Read the model definition and answer for the solid it produces. Units are mm, in the model's axes. A direction names the side the tool comes from. Coordinates: 2 decimals unless noted, no trailing zeros. Loops run counter-clockwise (first coordinate to the right, second up) from the corner with the lowest first, then second, coordinate; pieces in that order, holes last. Notation, with made-up numbers: (50.25, 9) -> (71.25, 9) arc R6 ccw to (71.25, 14) -> close; hole circle Ø8 at (82.25, 38.5). An arc over 180 degrees is marked (long way). Answer as a JSON object with one key per item and string values. Group by question number.
Q1. Straight lines are drawn through the part: line 1 along X through (y, z) = (-15, 187); line 2 along X through (y, z) = (-0.5, 65.5); line 3 along Y through (x, z) = (12, 143). For each, find the intervals that lie inside material, in ascending order. Write a range as [from, to].
Q2. The part is cut by section B-B on z = 196.5. State how many separate pieces and enclosed holes the cut face has, and give its area (3 significant figures).
Q3. Determine the mould class of faces 1 (the flat face through (45, -13, 125)), 2 (the cylindrical face through (41.5, -19.07, 125.22)) for opening direction Y: released by +Y, released by -Y, zero draft, split by the parting line, or undercut.
Q4. Each of these flat-tipped pins is pushed along its axis until it touches: P1, Ø1.5, axis at x = 21.5, y = -9, coming from the +Z side; P2, Ø2.5, axis at x = 24.5, z = 188.5, coming from the -Y side; P3, Ø4, axis at x = -34.5, y = -10.5, coming from the +Z side. Where does it stop, or does it pass through?
Q5. The part is cut by section A-A on x = 6. Write down the section's boundary in (y, z).
Q6. For faces 3 (the flat face through (-43, -4.1, 125)), 4 (the flat face through (43, -4.1, 125)), 5 (the flat face through (15.5, 0, 125)), determine the directions among +Z, -Z, +X, -X, +Y, -Y from which every point of the face is accessible in a straight line to the end or side of a thin tool.
from build123d import *

# Parameters (mm, degrees)
BOSS_EXTRUDE1_DEPTH = 254


with BuildPart() as part:
    # Sketch1 → Boss-Extrude1 (new body)
    with BuildSketch(Plane(origin=(0, 0, 0), x_dir=(-1, 0, 0), z_dir=(0, 0, -1))):
        Polygon((-26.6, 22.5), (-45, 22.5), (-45, 4.1), (-40.5, 4.1), (-40.5, 6.8), (-32, 6.8), (-29.7, 4.5), (-29.7, -4.5), (-32, -6.8), (-40.5, -6.8), (-40.5, -4.1), (-45, -4.1), (-45, -22.5), (-26.6, -22.5), (-26.6, -18), (-29.3, -18), (-29.3, -9.5), (-27, -7.2), (-18, -7.2), (-15.7, -9.5), (-15.7, -18), (-18.4, -18), (-18.4, -22.5), (18.4, -22.5), (18.4, -18), (15.7, -18), (15.7, -9.5), (18, -7.2), (27, -7.2), (29.3, -9.5), (29.3, -18), (26.6, -18), (26.6, -22.5), (45, -22.5), (45, -4.1), (40.5, -4.1), (40.5, -6.8), (32, -6.8), (29.7, -4.5), (29.7, 4.5), (32, 6.8), (40.5, 6.8), (40.5, 4.1), (45, 4.1), (45, 22.5), (26.6, 22.5), (26.6, 18), (29.3, 18), (29.3, 9.5), (27, 7.2), (18, 7.2), (15.7, 9.5), (15.7, 18), (18.4, 18), (18.4, 22.5), (-18.4, 22.5), (-18.4, 18), (-15.7, 18), (-15.7, 9.5), (-18, 7.2), (-27, 7.2), (-29.3, 9.5), (-29.3, 18), (-26.6, 18), align=None)
        with BuildLine():
            Line((14.914213713, -7.157382523), (14.285798144, -7.785798093))
            ThreePointArc((14.285798144, -7.785798093), (13.852252641, -8.434644791), (13.700011706, -9.200011655))
            Line((13.700011706, -9.200011655), (13.700011706, -20.5))
            Line((13.700011706, -20.5), (-13.700011706, -20.5))
            Line((-13.700011706, -20.5), (-13.700011706, -9.200011568))
            ThreePointArc((-13.700011706, -9.200011568), (-13.852252624, -8.434644744), (-14.285798082, -7.785798067))
            Line((-14.285798082, -7.785798067), (-14.914213624, -7.15738247))
            ThreePointArc((-14.914213624, -7.15738247), (-15.347759082, -6.508535794), (-15.5, -5.74316897))
            Line((-15.5, -5.74316897), (-15.5, 5.7431692))
            ThreePointArc((-15.5, 5.7431692), (-15.347759065, 6.508536064), (-14.914213562, 7.157382762))
            Line((-14.914213562, 7.157382762), (-14.285798144, 7.78579818))
            ThreePointArc((-14.285798144, 7.78579818), (-13.852252641, 8.434644878), (-13.700011706, 9.200011743))
            Line((-13.700011706, 9.200011743), (-13.700011706, 20.5))
            Line((-13.700011706, 20.5), (13.700011706, 20.5))
            Line((13.700011706, 20.5), (13.700011706, 9.200011728))
            ThreePointArc((13.700011706, 9.200011728), (13.852252624, 8.434644904), (14.285798082, 7.785798227))
            Line((14.285798082, 7.785798227), (14.914213775, 7.157382479))
            ThreePointArc((14.914213775, 7.157382479), (15.347759233, 6.508535803), (15.500000151, 5.743168979))
            Line((15.500000151, 5.743168979), (15.500000151, -5.743168961))
            ThreePointArc((15.500000151, -5.743168961), (15.347759216, -6.508535826), (14.914213713, -7.157382523))
        make_face(mode=Mode.SUBTRACT)
        with BuildLine():
            Line((43, 15.5), (43, 8.799988823))
            Line((43, 8.799988823), (36.300017792, 8.799988823))
            ThreePointArc((36.300017792, 8.799988823), (32.764483886, 10.264454917), (31.300017792, 13.799988823))
            Line((31.300017792, 13.799988823), (31.300017792, 20.5))
            Line((31.300017792, 20.5), (38, 20.5))
            ThreePointArc((38, 20.5), (41.535533906, 19.035533906), (43, 15.5))
        make_face(mode=Mode.SUBTRACT)
        with BuildLine():
            Line((-36.300017792, 8.799988823), (-43, 8.799988823))
            Line((-43, 8.799988823), (-43, 15.5))
            ThreePointArc((-43, 15.5), (-41.535533906, 19.035533906), (-38, 20.5))
            Line((-38, 20.5), (-31.300017792, 20.5))
            Line((-31.300017792, 20.5), (-31.300017792, 13.799988823))
            ThreePointArc((-31.300017792, 13.799988823), (-32.764483886, 10.264454917), (-36.300017792, 8.799988823))
        make_face(mode=Mode.SUBTRACT)
        with BuildLine():
            Line((-43, -15.5), (-43, -8.7999878))
            Line((-43, -8.7999878), (-36.300017792, -8.7999878))
            ThreePointArc((-36.300017792, -8.7999878), (-32.764483886, -10.264453894), (-31.300017792, -13.7999878))
            Line((-31.300017792, -13.7999878), (-31.300017792, -20.5))
            Line((-31.300017792, -20.5), (-38, -20.5))
            ThreePointArc((-38, -20.5), (-41.535533906, -19.035533906), (-43, -15.5))
        make_face(mode=Mode.SUBTRACT)
        with BuildLine():
            Line((36.300017792, -8.7999878), (43, -8.7999878))
            Line((43, -8.7999878), (43, -15.5))
            ThreePointArc((43, -15.5), (41.535533906, -19.035533906), (38, -20.5))
            Line((38, -20.5), (31.300017792, -20.5))
            Line((31.300017792, -20.5), (31.300017792, -13.7999878))
            ThreePointArc((31.300017792, -13.7999878), (32.764483886, -10.264453894), (36.300017792, -8.7999878))
        make_face(mode=Mode.SUBTRACT)
        with BuildLine():
            Line((-20.651475745, 3.262737818), (-19.318019484, 4.59619408))
            Line((-19.318019484, 4.59619408), (-17.903805921, 3.181980517))
            Line((-17.903805921, 3.181980517), (-19.237262182, 1.848524255))
            ThreePointArc((-19.237262182, 1.848524255), (-18.750000002, 0), (-19.237262183, -1.848524255))
            Line((-19.237262183, -1.848524255), (-17.903805921, -3.181980517))
            Line((-17.903805921, -3.181980517), (-19.318019483, -4.596194079))
            Line((-19.318019483, -4.596194079), (-20.651475745, -3.262737818))
            ThreePointArc((-20.651475745, -3.262737818), (-22.5, -3.749999998), (-24.348524255, -3.262737818))
            Line((-24.348524255, -3.262737818), (-25.681980515, -4.596194078))
            Line((-25.681980515, -4.596194078), (-27.096194078, -3.181980516))
            Line((-27.096194078, -3.181980516), (-25.762737818, -1.848524255))
            ThreePointArc((-25.762737818, -1.848524255), (-26.249999999, 0), (-25.762737818, 1.848524255))
            Line((-25.762737818, 1.848524255), (-27.096194079, 3.181980517))
            Line((-27.096194079, 3.181980517), (-25.681980517, 4.596194079))
            Line((-25.681980517, 4.596194079), (-24.348524255, 3.262737818))
            ThreePointArc((-24.348524255, 3.262737818), (-22.5, 3.749999999), (-20.651475745, 3.262737818))
        make_face(mode=Mode.SUBTRACT)
        with BuildLine():
            Line((27.096194079, 3.181980516), (25.762737818, 1.848524255))
            ThreePointArc((25.762737818, 1.848524255), (26.249999999, 0), (25.762737818, -1.848524255))
            Line((25.762737818, -1.848524255), (27.09619408, -3.181980517))
            Line((27.09619408, -3.181980517), (25.681980518, -4.596194079))
            Line((25.681980518, -4.596194079), (24.348524256, -3.262737818))
            ThreePointArc((24.348524256, -3.262737818), (22.500000001, -3.749999999), (20.651475745, -3.262737818))
            Line((20.651475745, -3.262737818), (19.318019485, -4.596194078))
            Line((19.318019485, -4.596194078), (17.903805922, -3.181980515))
            Line((17.903805922, -3.181980515), (19.237262182, -1.848524255))
            ThreePointArc((19.237262182, -1.848524255), (18.750000002, 0), (19.237262182, 1.848524255))
            Line((19.237262182, 1.848524255), (17.903805921, 3.181980516))
            Line((17.903805921, 3.181980516), (19.318019483, 4.596194079))
            Line((19.318019483, 4.596194079), (20.651475745, 3.262737817))
            ThreePointArc((20.651475745, 3.262737817), (22.5, 3.749999998), (24.348524255, 3.262737818))
            Line((24.348524255, 3.262737818), (25.681980517, 4.596194079))
            Line((25.681980517, 4.596194079), (27.096194079, 3.181980516))
        make_face(mode=Mode.SUBTRACT)
    extrude(amount=-BOSS_EXTRUDE1_DEPTH)


solid = part.part
Final values:
{
 "1": {"line 1": "x = [-45, -43], [-31.3, -29.3], [-15.7, -13.7], [13.7, 15.7], [29.3, 31.3], [43, 45]", "line 2": "x = [-29.7, -26.22], [-18.78, -15.5], [15.5, 18.78], [26.22, 29.7]", "line 3": "y = [-22.5, -20.5], [20.5, 22.5]"},
 "2": {"separate pieces": "1", "enclosed holes": "7", "area": "1,180 mm2"},
 "3": {"face 1": "zero draft", "face 2": "undercut"},
 "4": {"P1": "passes through", "P2": "stops at y = -7.2", "P3": "stops at z = 254"},
 "5": {"outline": "(-22.5, 0) -> (-20.5, 0) -> (-20.5, 254) -> (-22.5, 254) -> close; (20.5, 0) -> (22.5, 0) -> (22.5, 254) -> (20.5, 254) -> close"},
 "6": {"face 3": "+Z, -Z, -X", "face 4": "+Z, -Z, +X", "face 5": "+Z, -Z"}
}
